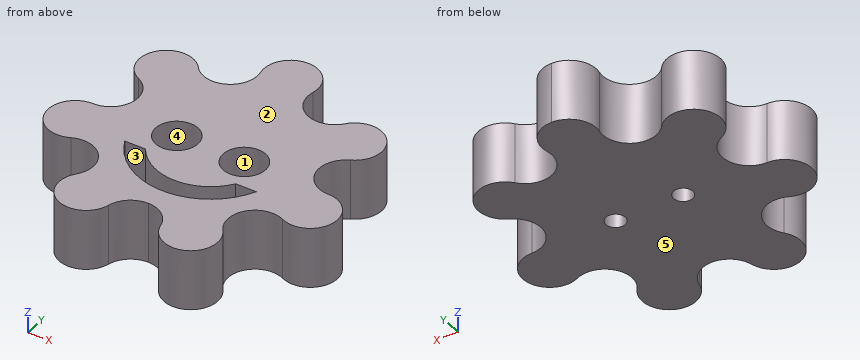
from build123d import *

# Parameters (mm, degrees)
PAD004_DEPTH         = 5
SKETCH012_R          = 0.8
POCKET006_DEPTH      = 67.792744
POCKET006_DEPTH_BACK = 72.792744
SKETCH013_R          = 1.75
POCKET007_DEPTH      = 70.792744
POCKET009_DEPTH      = 5


with BuildPart() as part:
    # Sketch011 (on DatumPlane) → Pad004 (new body)
    with BuildSketch(Plane.XY.offset(6)):
        with BuildLine():
            ThreePointArc((0, 12.225209), (-1.739739, 11.387395), (-2.169419, 9.504844))
            ThreePointArc((-6.078576, 7.622293), (-3.373355, 7.004844), (-2.169419, 9.504844))
            ThreePointArc((-6.078576, 7.622293), (-9.558054, 7.622293), (-8.783797, 4.230054))
            ThreePointArc((-9.749279, 0), (-7.57986, 1.730054), (-8.783797, 4.230054))
            ThreePointArc((-9.749279, 0), (-11.918698, -2.720365), (-8.783797, -4.230054))
            ThreePointArc((-6.078576, -7.622293), (-6.078576, -4.847503), (-8.783797, -4.230054))
            ThreePointArc((-6.078576, -7.622293), (-5.30432, -11.014533), (-2.169419, -9.504844))
            ThreePointArc((0, -7.774791), (-1.387395, -8.260261), (-2.169419, -9.504844))
            Line((0, 12.225209), (0, -7.774791))
        make_face()
    pad004 = extrude(amount=PAD004_DEPTH)

    # Mirrored003: Pad004 across Sketch011 V_Axis
    add(pad004.mirror(Plane(origin=(0, 0, 6), x_dir=(0, 0, 1), z_dir=(1, 0, 0))))

    # Sketch012 (on DatumPlane) → Pocket006 (cut, two sides)
    with BuildSketch(Plane.XY.offset(6)) as pocket006_sk:
        with Locations((-2.8, 0)):
            Circle(SKETCH012_R)
    pocket006 = extrude(amount=-POCKET006_DEPTH, mode=Mode.SUBTRACT) + extrude(pocket006_sk.sketch, amount=POCKET006_DEPTH_BACK, mode=Mode.SUBTRACT)

    # Sketch013 (on DatumPlane) → Pocket007 (cut, through all)
    with BuildSketch(Plane.XY.offset(8)):
        with Locations((-2.8, 0)):
            Circle(SKETCH013_R)
    pocket007 = extrude(amount=POCKET007_DEPTH, mode=Mode.SUBTRACT)

    # Mirrored004: Pocket006, Pocket007 across Sketch012 V_Axis
    add(pocket006.mirror(Plane(origin=(0, 0, 6), x_dir=(0, 0, 1), z_dir=(1, 0, 0))), mode=Mode.SUBTRACT)
    add(pocket007.mirror(Plane(origin=(0, 0, 6), x_dir=(0, 0, 1), z_dir=(1, 0, 0))), mode=Mode.SUBTRACT)

    # Sketch014 (on DatumPlane) → Pocket009 (cut)
    with BuildSketch(Plane.XY.offset(8)):
        with BuildLine():
            ThreePointArc((-5.454356, -2.5), (0, -6), (5.454356, -2.5))
            Line((3.741657, -2.5), (5.454356, -2.5))
            ThreePointArc((-3.741657, -2.5), (0, -4.5), (3.741657, -2.5))
            Line((-5.454356, -2.5), (-3.741657, -2.5))
        make_face()
    extrude(amount=POCKET009_DEPTH, mode=Mode.SUBTRACT)


solid = part.part
Here's how the part is built. I have some questions about the finished solid (model axes, mm). Face numbers are marked on the shaded views. A direction names the side the tool comes from. Round coordinates to 2 decimals unless told otherwise and drop trailing zeros. Order: outer loops, then holes, each group sorted by start corner. A loop starts at its lowest first (then second) coordinate and runs counter-clockwise, first axis right, second up. Notation, with made-up numbers: M -19.5,36 L 34.5,36 A30 cw 34.5,71 Z; hole C -37,40 d1. An arc over 180 degrees is marked long. Return JSON: item names as keys, results as strings. Group by question number.
1. If we section it at C-C on z = 10.15: List the corners of the cut face in (x, y) for me.
2. If we section it at A-A on y = -9: List the corners of the cut face in (x, z) for me.
3. On a 3-axis mill with a long thin cutter (end or side, diameter ignored), from which of +Z, -Z, +X, -X, +Y, -Y can I reach the whole of each face in a straight line? I mean the marked faces 1 and 2. Say none if no direction works.
4. I'm going to push flat-ended pins straight in: pin 1 Ø2 at (x, y) = (-2.8, 0) entering from +Z; pin 2 Ø1.5 at (x, z) = (-5, 9.5) entering from +Y; pin 3 Ø3 at (y, z) = (7.5, 10) entering from +X. Where does each tip first touch, or does it pass through?
5. Please list where these lines run through material, in increasing order: probe 1 along X at (y, z) = (7.5, 9.05); probe 2 along Y at (x, z) = (-2.8, 9.4); probe 3 along Y at (x, z) = (3, 9.8).
6. If we mould it in two halves opening along Y, with no side actions, what happens to the marked faces 3, 4 and 5? For each: pulls with the +Y half, pulls with the -Y half, needs draft (parallel to the pull), parting line crosses it, or undercut.
7. If we section it at B-B on x = 0.5: List the corners of the cut face in (y, z) for me, then the cut area to 3 significant figures.
8. If we section it at D-D on x = -2.8: List the corners of the cut face in (y, z) for me, then the cut area to 3 significant figures.
Reply:
{
 "1": {"outline": "M -9.75,0 A2.23 ccw long -8.78,-4.23 A2.23 cw -6.08,-7.62 A2.23 ccw long -2.17,-9.5 A2.23 cw 2.17,-9.5 A2.23 ccw long 6.08,-7.62 A2.23 cw 8.78,-4.23 A2.23 ccw long 9.75,0 A2.23 cw 8.78,4.23 A2.23 ccw long 6.08,7.62 A2.23 cw 2.17,9.5 A2.23 ccw long -2.17,9.5 A2.23 cw -6.08,7.62 A2.23 ccw long -8.78,4.23 A2.23 cw Z; hole M -5.45,-2.5 A6 ccw 5.45,-2.5 L 3.74,-2.5 A4.5 cw -3.74,-2.5 Z; hole C -2.8,0 d3.5; hole C 2.8,0 d3.5"},
 "2": {"outline": "M -6.56,6 L -1.99,6 L -1.99,11 L -6.56,11 Z; M 1.99,6 L 6.56,6 L 6.56,11 L 1.99,11 Z"},
 "3": {"face 1": "+Z", "face 2": "+Z, +X, -X, +Y, -Y"},
 "4": {"pin 1": "z = 8", "pin 2": "y = 7.29", "pin 3": "x = 10.04"},
 "5": {"probe 1": "-9.65 to -5.97, -2.7 to 2.7, 5.97 to 9.65", "probe 2": "-10.62 to -5.31, -3.52 to -1.75, 1.75 to 7.4", "probe 3": "-10.79 to -5.2, -3.35 to -1.74, 1.74 to 7.23"},
 "6": {"face 3": "undercut", "face 4": "undercut", "face 5": "needs draft"},
 "7": {"outline": "M -7.83,6 L 12.17,6 L 12.17,11 L -4.47,11 L -4.47,8 L -5.98,8 L -5.98,11 L -7.83,11 Z", "area": "95.5 mm^2"},
 "8": {"outline": "M -10.62,6 L -0.8,6 L -0.8,8 L -1.75,8 L -1.75,11 L -3.52,11 L -3.52,8 L -5.31,8 L -5.31,11 L -10.62,11 Z; M 0.8,6 L 7.4,6 L 7.4,11 L 1.75,11 L 1.75,8 L 0.8,8 Z", "area": "71.0 mm^2"}
}
